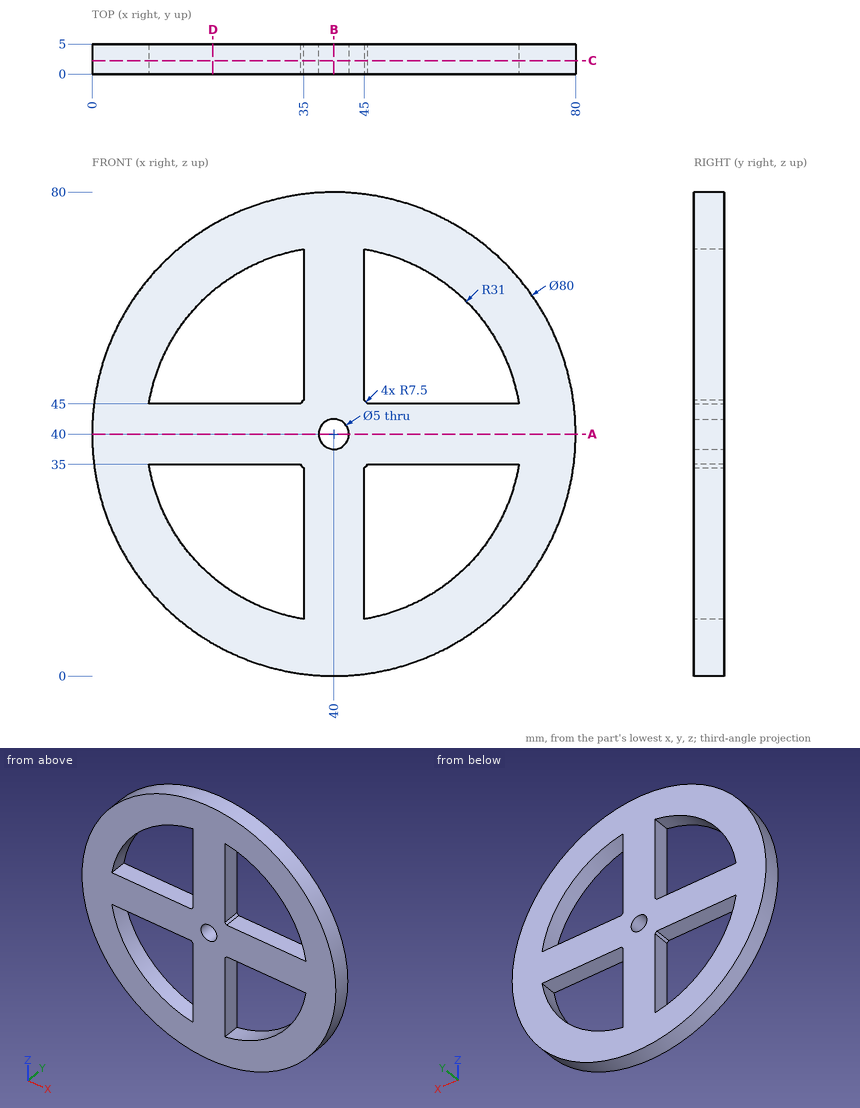
Geometry: see drawing. Coordinates: mm, zero at the bounding-box minimum. Give positions to 0.01 mm unless a question says otherwise; leave off trailing zeros. Loops run counter-clockwise (first coordinate to the right, second up) from the corner with the lowest first, then second, coordinate; pieces in that order, holes last. Notation, with made-up numbers: M 68,-28 L 78,-28 A34 cw 78,3 Z; hole C 80,-10 d4. An arc over 180 degrees is marked long. Use one line per item in the form item = value.
1. Section query D-D, the plane x = 20. Return the cut outline in (y, z), and give its area (3 significant figures).
Numbers:
outline = M 0,5.36 L 5,5.36 L 5,16.31 L 0,16.31 Z; M 0,35 L 5,35 L 5,45 L 0,45 Z; M 0,63.69 L 5,63.69 L 5,74.64 L 0,74.64 Z
area = 160 mm²
2. Section query B-B, the plane x = 40. Return the cut outline in (y, z).
Numbers:
outline = M 0,0 L 5,0 L 5,37.5 L 0,37.5 Z; M 0,42.5 L 5,42.5 L 5,80 L 0,80 Z
3. Line query: L1, parallel to Z at x = 40, y = 3; L2, parallel to Z at x = 23, y = 3.9; L3, parallel to X at y = 0.7, z = 31.5. Output: solid intervals per line, ascending.
Numbers:
L1 = 0 to 37.5, 42.5 to 80
L2 = 3.79 to 14.08, 35 to 45, 65.92 to 76.21
L3 = 0.91 to 10.19, 35 to 45, 69.81 to 79.09
4. Section query A-A, the plane z = 40. Return the cut outline in (x, y).
Numbers:
outline = M 0,0 L 37.5,0 L 37.5,5 L 0,5 Z; M 42.5,0 L 80,0 L 80,5 L 42.5,5 Z
5. First-contact query: pin 1 (1.5 mm diameter, centred on x = 62, y = 3.5, fed in from +Z); pin 2 (1.5 mm diameter, centred on y = 2.5, z = 64.5, fed in from -X); pin 3 (1.5 mm diameter, centred on y = 2, z = 20.5, fed in from -X). Flat tips, straight axial feed; report the tip coordinate or a pass-through.
Numbers:
pin_1 = 73.89
pin_2 = 7.81
pin_3 = 4.67
6. Section query C-C, the plane y = 2.25. Return the cut outline in (x, z).
Numbers:
outline = C 40,40 d80; hole M 9.41,35 A31 ccw 35,9.41 L 35,34.41 A7.5 cw 34.41,35 Z; hole M 9.41,45 L 34.41,45 A7.5 cw 35,45.59 L 35,70.59 A31 ccw Z; hole C 40,40 d5; hole M 45,9.41 A31 ccw 70.59,35 L 45.59,35 A7.5 cw 45,34.41 Z; hole M 45,45.59 A7.5 cw 45.59,45 L 70.59,45 A31 ccw 45,70.59 Z
